from build123d import *

# Parameters (mm, degrees)
BOSS_EXTRUDE1_DEPTH = 1.5875
SKETCH2_R           = 3.175
BOSS_EXTRUDE2_DEPTH = 19.05
SKETCH3_R           = 2.0574
CUT_EXTRUDE1_DEPTH  = 6.35


with BuildPart() as part:
    # Sketch1 → Boss-Extrude1 (new body)
    with BuildSketch(Plane(origin=(0, 0, 0), x_dir=(1, 0, 0), z_dir=(0, 1, 0))):
        Polygon((4.7625, -1.972692091), (4.7625, 1.972692091), (1.972692091, 4.7625), (-1.972692091, 4.7625), (-4.7625, 1.972692091), (-4.7625, -1.972692091), (-1.972692091, -4.7625), (1.972692091, -4.7625), align=None)
    extrude(amount=BOSS_EXTRUDE1_DEPTH)

    # Sketch2 → Boss-Extrude2 (add)
    with BuildSketch(Plane(origin=(0, 1.5875, 0), x_dir=(1, 0, 0), z_dir=(0, 1, 0))):
        with Locations(Location((0, 0, 0), (0, 0, 90))):
            Circle(SKETCH2_R)
    extrude(amount=BOSS_EXTRUDE2_DEPTH)

    # Sketch3 → Cut-Extrude1 (cut)
    with BuildSketch(Plane(origin=(0, 20.6375, 0), x_dir=(1, 0, 0), z_dir=(0, 1, 0))):
        with Locations(Location((0, 0, 0), (0, 0, 270))):
            Circle(SKETCH3_R)
    extrude(amount=-CUT_EXTRUDE1_DEPTH, mode=Mode.SUBTRACT)


solid = part.part
Geometry check sheet. Reference: the model listing, model coordinates, mm. A direction names the side the tool comes from. Coordinates: 2 decimals unless noted, no trailing zeros. Write each loop counter-clockwise with the first axis right and the second up, starting at its lowest first coordinate (ties: lowest second). Pieces come first, ordered by that corner, then holes. Notation, with made-up numbers: (77.5, 28) -> (112.5, 28) arc R25 ccw to (112.5, 52) -> close; hole circle Ø11 at (38.5, 81). An arc over 180 degrees is marked (long way). One line per question, with ' | ' between items.
1. Cross-section at D-D on y = 2.75. Record the cut outline in (x, z) (3 decimals), and give its area (3 significant figures).
Answers:
outline: circle Ø6.35 at (0, 0) | area: 31.7 mm²
2. Draft check along X on faces 3 (the cylindrical face through (-0.79, 17.51, 1.9)), 4 (the flat face through (3.387, 0.783, -3.348)), 5 (the flat face through (0, 0, 0)). Enter one of: +X half, -X half, draft (parallel to the pull), parting line (faces both ways), or undercut.
Answers:
face 3: undercut | face 4: +X half | face 5: draft
3. Depth check by flat-ended pin: pin 1 Ø1.5 at (x, z) = (-3, -3.5) entering from +Y; pin 2 Ø3 at (x, y) = (1, 10.5) entering from +Z (3 decimals); pin 3 Ø2 at (x, z) = (-0.5, 1) entering from +Y. Enter the tip coordinate at first touch or a pass-through.
Answers:
pin 1: stops at y = 1.59 | pin 2: stops at z = 3.175 | pin 3: stops at y = 20.64
4. Cross-section at C-C on y = 18.5. Record the cut outline in (x, z) (3 decimals), and give its area (3 significant figures).
Answers:
outline: circle Ø6.35 at (0, 0); hole circle Ø4.115 at (0, 0) | area: 18.4 mm²
5. Set-up check for faces 1 (the flat face through (0, 1, -4.762)), 2 (the cylindrical face through (1.93, 10.98, 2.52)): record each of +Z, -Z, +X, -X, +Y, -Y from which the full face is reachable in a straight line by a thin tool's end or side.
Answers:
face 1: -Z, +X, -X, +Y, -Y | face 2: +Y
6. Cross-section at B-B on z = 0. Record the cut outline in (x, y) (1 decimal), and give its area (3 significant figures).
Answers:
outline: (-4.8, 0) -> (4.8, 0) -> (4.8, 1.6) -> (3.2, 1.6) -> (3.2, 20.6) -> (2.1, 20.6) -> (2.1, 14.3) -> (-2.1, 14.3) -> (-2.1, 20.6) -> (-3.2, 20.6) -> (-3.2, 1.6) -> (-4.8, 1.6) -> close | area: 110 mm²
7. Thickness scan on probe 1 along X at (y, z) = (17, 0) (3 decimals); probe 2 along Y at (x, z) = (3.5, 1.5); probe 3 along X at (y, z) = (16, -1.25). Record the ranges inside material, lowest first. Write a range as from..to.
Answers:
probe 1: x = -3.175..-2.057, 2.057..3.175 | probe 2: y = 0..1.59 | probe 3: x = -2.92..-1.63, 1.63..2.92
8. Cross-section at A-A on x = 0. Record the cut outline in (y, z) (1 decimal), and give its area (3 significant figures).
Answers:
outline: (0, -4.8) -> (1.6, -4.8) -> (1.6, -3.2) -> (20.6, -3.2) -> (20.6, -2.1) -> (14.3, -2.1) -> (14.3, 2.1) -> (20.6, 2.1) -> (20.6, 3.2) -> (1.6, 3.2) -> (1.6, 4.8) -> (0, 4.8) -> close | area: 110 mm²
